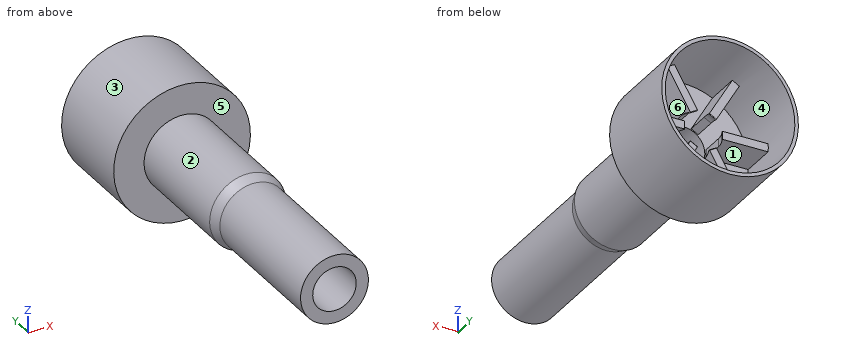
from build123d import *

# Parameters (mm, degrees)
BOSS_EXTRUDE1_DEPTH      = 0.4
FILLET1_R                = 0.05
CIRPATTERN1_COUNT        = 6
FILLET1_OF_CIRPATTERN1_R = 0.05


with BuildPart() as part:
    # Sketch1 → Revolve1 (revolve)
    with BuildSketch(Plane.XY, mode=Mode.PRIVATE) as revolve1_sk:
        Polygon((-6.4, 36.5), (-6.4, 28.2), (-2.1, 28.2), (-2.1, 24), (-1.5, 24), (-1.5, 23), (-2.15, 23), (-2.15, 0), (-3.35, 0), (-3.35, 14.401009032), (-3.75, 15.5), (-3.75, 27.2), (-6.75, 27.2), (-6.75, 36.5), align=None)
    revolve(revolve1_sk.sketch.rotate(Axis((0, 0, 0), (0, 1, 0)), 270), axis=Axis((0, 0, 0), (0, 1, 0)))

    # Sketch3 → Boss-Extrude1 (add, symmetric)
    with BuildSketch(Plane.XY):
        with BuildLine():
            Line((-2.2, 28.2), (-2.2, 30.5))
            ThreePointArc((-2.2, 30.5), (-2.097563242, 31.156220237), (-1.8, 31.75))
            Line((-1.8, 31.75), (-6.4, 31.75))
            Line((-6.4, 31.75), (-6.4, 28.2))
            Line((-6.4, 28.2), (-2.2, 28.2))
        make_face()
    boss_extrude1 = extrude(amount=BOSS_EXTRUDE1_DEPTH, both=True)

    # Fillet1
    fillet1_edges = [part.edges().sort_by_distance(p)[0] for p in [
        (-1.8, 31.75, 0),
    ]]
    fillet(fillet1_edges, radius=FILLET1_R)

    # CirPattern1: Boss-Extrude1 ×6 about axis
    cirpattern1_axis = Axis((0, 0, 0), (0, 1, 0))
    for i in range(1, CIRPATTERN1_COUNT):
        add(boss_extrude1.rotate(cirpattern1_axis, i * 360 / CIRPATTERN1_COUNT))

    # Fillet1 of CirPattern1
    fillet1_of_cirpattern1_edges = [part.edges().sort_by_distance(p)[0] for p in [
        (-0.9, 31.75, 1.558845727),
        (0.9, 31.75, 1.558845727),
        (1.8, 31.75, 0),
        (0.9, 31.75, -1.558845727),
        (-0.9, 31.75, -1.558845727),
    ]]
    fillet(fillet1_of_cirpattern1_edges, radius=FILLET1_OF_CIRPATTERN1_R)


solid = part.part
Can you work these out from the model? Positions are in its coordinate system, mm. Face numbers are marked on the shaded views. A direction names the side the tool comes from. Coordinates: 2 decimals unless noted, no trailing zeros. Write each loop counter-clockwise with the first axis right and the second up, starting at its lowest first coordinate (ties: lowest second). Pieces come first, ordered by that corner, then holes. Notation, with made-up numbers: (71.25, -18.75) - (100.25, -18.75) arc R21 cw to (100.25, 3.25) - close; hole circle Ø2 at (5.5, 44). An arc over 180 degrees is marked (long way). Return JSON: item names as keys, results as strings. Group by question number.
Item 1: Please list where these lines run through material, in increasing order: probe 1 along X at (y, z) = (10.5, 0); probe 2 along X at (y, z) = (26.2, 0); probe 3 along Y at (x, z) = (-2.25, 1.75).
Item 2: I'm going to push flat-ended pins straight in: pin 1 Ø5 at (x, z) = (-1.5, -5) entering from +Y; pin 2 Ø3.5 at (x, z) = (0, 0) entering from +Y; pin 3 Ø1.8 at (x, y) = (-4, 30) entering from +Z; pin 4 Ø1.5 at (x, z) = (2, 2.5) entering from +Y. Where does each tip first touch, or does it pass through?
Item 3: We'd pull the mould along Z, two halves only. Please class the marked faces 3, 4, 5 and 6: pulls with the +Z half, pulls with the -Z half, needs draft (parallel to the pull), parting line crosses it, or undercut.
Item 4: If we section it at C-C (z = 4.5): Write out the boundary of the cut face in (x, y).
Item 5: If we section it at B-B (y = 29.5): Write out the boundary of the cut face in (x, z).
Item 6: If we section it at D-D (x = -5.75): Write out the boundary of the cut face in (y, z), then the cut area to 3 significant figures.
Item 7: Which directions (+Z, -Z, +X, -X, +Y, -Y) give clear straight access to the entire face, cutting with the end or side of a thin tool? Please do the marked faces 1 and 2.
Item 8: If we section it at A-A (x = 0): Write out the boundary of the cut face in (y, z).
Return value:
{
 "1": {"probe 1": "x = -3.35 to -2.15, 2.15 to 3.35", "probe 2": "x = -3.75 to -2.1, 2.1 to 3.75", "probe 3": "y = 0 to 28.2"},
 "2": {"pin 1": "stops at y = 36.5", "pin 2": "stops at y = 24", "pin 3": "stops at z = 6", "pin 4": "stops at y = 31.75"},
 "3": {"face 3": "parting line crosses it", "face 4": "undercut", "face 5": "needs draft", "face 6": "undercut"},
 "4": {"outline": "(-5.03, 27.2) - (5.03, 27.2) - (5.03, 36.5) - (4.55, 36.5) - (4.55, 28.2) - (3.06, 28.2) - (3.06, 31.75) - (2.14, 31.75) - (2.14, 28.2) - (-2.14, 28.2) - (-2.14, 31.75) - (-3.06, 31.75) - (-3.06, 28.2) - (-4.55, 28.2) - (-4.55, 36.5) - (-5.03, 36.5) - close"},
 "5": {"outline": "circle Ø13.5 at (0, 0); hole (-6.39, -0.4) arc R6.4 ccw to (-3.54, -5.33) - (-1.45, -1.71) - (-0.75, -2.11) - (-2.85, -5.73) arc R6.4 ccw to (2.85, -5.73) - (0.75, -2.11) - (1.45, -1.71) - (3.54, -5.33) arc R6.4 ccw to (6.39, -0.4) - (2.2, -0.4) - (2.2, 0.4) - (6.39, 0.4) arc R6.4 ccw to (3.54, 5.33) - (1.45, 1.71) - (0.75, 2.11) - (2.85, 5.73) arc R6.4 ccw to (-2.85, 5.73) - (-0.75, 2.11) - (-1.45, 1.71) - (-3.54, 5.33) arc R6.4 ccw to (-6.39, 0.4) - (-2.2, 0.4) - (-2.2, -0.4) - close"},
 "6": {"outline": "(27.2, -3.54) - (36.5, -3.54) - (36.5, -2.81) - (28.2, -2.81) - (28.2, -0.4) - (31.75, -0.4) - (31.75, 0.4) - (28.2, 0.4) - (28.2, 2.81) - (36.5, 2.81) - (36.5, 3.54) - (27.2, 3.54) - close", "area": "22.0 mm^2"},
 "7": {"face 1": "+Y", "face 2": "-Y"},
 "8": {"outline": "(0, -3.35) - (14.4, -3.35) - (15.5, -3.75) - (27.2, -3.75) - (27.2, -6.75) - (36.5, -6.75) - (36.5, -6.4) - (28.2, -6.4) - (28.2, -2.1) - (24, -2.1) - (24, -1.5) - (23, -1.5) - (23, -2.15) - (0, -2.15) - close; (0, 2.15) - (23, 2.15) - (23, 1.5) - (24, 1.5) - (24, 2.1) - (28.2, 2.1) - (28.2, 6.4) - (36.5, 6.4) - (36.5, 6.75) - (27.2, 6.75) - (27.2, 3.75) - (15.5, 3.75) - (14.4, 3.35) - (0, 3.35) - close"}
}
